Check sheet for the modelled part. Datum: model origin and axes. Units: mm. Give positions to 0.01 mm unless a question says otherwise; leave off trailing zeros. Write each loop counter-clockwise with the first axis right and the second up, starting at its lowest first coordinate (ties: lowest second). Pieces come first, ordered by that corner, then holes. Notation, with made-up numbers: (-12.5, 72.5) -> (11.5, 72.5) arc R18 cw to (11.5, 106.5) -> close; hole circle Ø8 at (-35, 3). An arc over 180 degrees is marked (long way). Return JSON: item names as keys, results as strings.
from build123d import *

# Parameters (mm, degrees)
F2_DEPTH = 50
F3_DEPTH = 1


with BuildPart() as f2:
    # F1 (on Top) → F2 (new body)
    with BuildSketch(Plane.XY):
        Polygon((1.74609, 3.024317), (-1.74609, 3.024317), (-3.492181, 0), (-1.74609, -3.024317), (1.74609, -3.024317), (3.492181, 0), align=None)
    extrude(amount=-F2_DEPTH)

    # F0 (on Right) → F3 (join)
    with BuildSketch(Plane.YZ):
        Polygon((-54.671764, 69.118708), (-54.671764, 0), (-8.214929, 0), (6.51529, 0), (56.088127, 0), (56.088127, 69.118708), align=None)
    extrude(amount=F3_DEPTH)


solid = f2.part
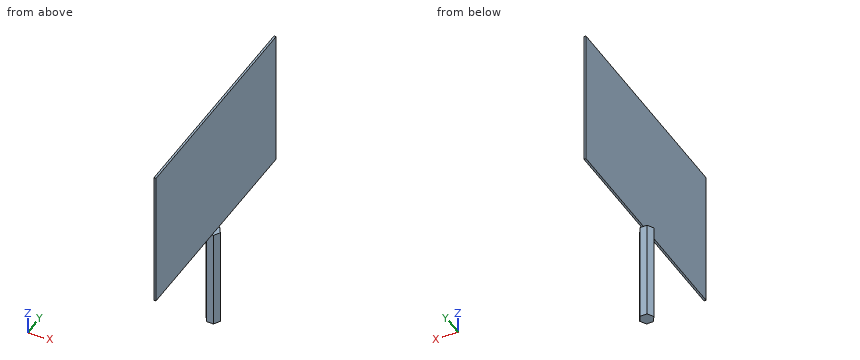
(1) Cross-section at A-A on z = -34.5. Enter the section's corners in (x, y).
Reply:
{"outline": "(-3.49, 0) -> (-1.75, -3.02) -> (1.75, -3.02) -> (3.49, 0) -> (1.75, 3.02) -> (-1.75, 3.02) -> close"}
(2) Cross-section at B-B on y = 34.5. Enter the section's corners in (x, z), then the cut area to 3 significant figures.
Reply:
{"outline": "(0, 0) -> (1, 0) -> (1, 69.12) -> (0, 69.12) -> close", "area": "69.1 mm^2"}
(3) Thickness scan on L1, parallel to Y at x = 2.5, z = -25; L2, parallel to X at y = -10, z = 50; L3, parallel to Y at x = -1.5, z = -27. Record the ranges inside material, lowest first.
Reply:
{"L1": "-1.72 to 1.72", "L2": "0 to 1", "L3": "-3.02 to 3.02"}
(4) Depth check by flat-ended pin: pin 1 Ø2 at (x, z) = (2.5, -12) entering from -Y; pin 2 Ø0.8 at (x, y) = (0.5, -38.5) entering from -Z; pin 3 Ø2 at (y, z) = (13.5, 54) entering from -X. Enter the tip coordinate at first touch or a pass-through.
Reply:
{"pin 1": "y = -3.02", "pin 2": "z = 0", "pin 3": "x = 0"}
(5) Cross-section at C-C on z = 60. Enter the section's corners in (x, y).
Reply:
{"outline": "(0, -54.67) -> (1, -54.67) -> (1, 56.09) -> (0, 56.09) -> close"}
